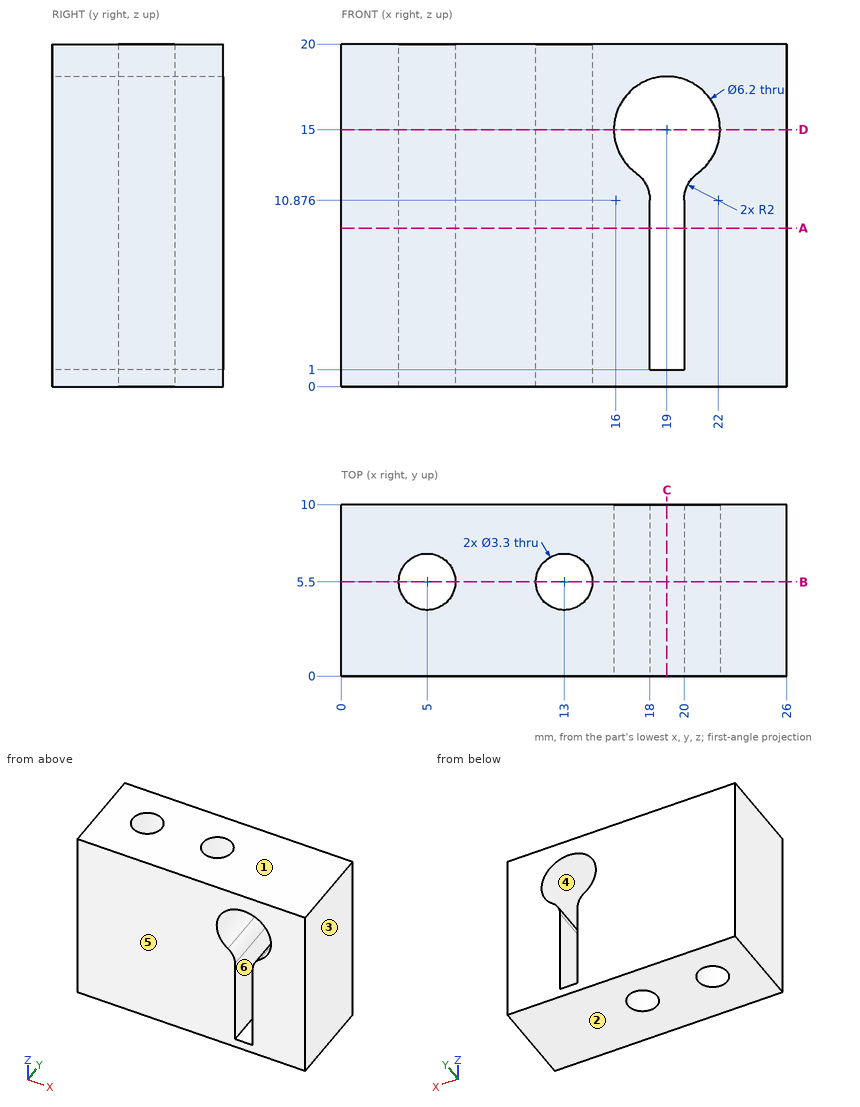
The figure shows three views and two pictorial views of one solid part (mm, origin at its lowest corner). Answer the questions. A direction names the side the tool comes from. Round coordinates to 2 decimals unless told otherwise and drop trailing zeros. Write each loop counter-clockwise with the first axis right and the second up, starting at its lowest first coordinate (ties: lowest second). Pieces come first, ordered by that corner, then holes. Notation, with made-up numbers: (-3.75, -24.5) -> (37.25, -24.5) arc R13 ccw to (37.25, -2.5) -> close; hole circle Ø9 at (51, -12). An arc over 180 degrees is marked (long way). Answer as a JSON object with one key per item and string values. Group by question number.
Q1. Determine the mould class of the marked faces 1, 2, 3 and 4 for opening direction Z: pulls with the +Z half, pulls with the -Z half, needs draft (parallel to the pull), parting line crosses it, or undercut.
Q2. Section A-A (z = 9.25) is taken. Write down the section's boundary in (x, y), plus the area to 3 significant figures.
Q3. Section B-B (y = 5.5) is taken. Write down the section's boundary in (x, z).
Q4. Section C-C (x = 19) is taken. Write down the section's boundary in (y, z).
Q5. Which of the six approach directions +Z, -Z, +X, -X, +Y, -Y give full straight-line access (tool end or side, diameter ignored) to the marked faces 5 and 6?
Q6. Straight lines are drawn through the part: line 1 along Y through (x, z) = (5, 5.25); line 2 along X through (y, z) = (7.5, 4.25); line 3 along X through (y, z) = (6, 12) (1 decimal). For each, find the intervals that lie inside material, in ascending order.
Q7. Section D-D (z = 15) is taken. Write down the section's boundary in (x, y), plus the area to 3 significant figures.
Check values:
{
 "1": {"face 1": "pulls with the +Z half", "face 2": "pulls with the -Z half", "face 3": "needs draft", "face 4": "undercut"},
 "2": {"outline": "(0, 0) -> (18, 0) -> (18, 10) -> (0, 10) -> close; (20, 0) -> (26, 0) -> (26, 10) -> (20, 10) -> close; hole circle Ø3.3 at (5, 5.5); hole circle Ø3.3 at (13, 5.5)", "area": "223 mm^2"},
 "3": {"outline": "(0, 0) -> (3.35, 0) -> (3.35, 20) -> (0, 20) -> close; (6.65, 0) -> (11.35, 0) -> (11.35, 20) -> (6.65, 20) -> close; (14.65, 0) -> (26, 0) -> (26, 20) -> (14.65, 20) -> close; hole (17.18, 12.49) arc R2 cw to (18, 10.88) -> (18, 1) -> (20, 1) -> (20, 10.88) arc R2 cw to (20.82, 12.49) arc R3.1 ccw (long way) to start"},
 "4": {"outline": "(0, 0) -> (10, 0) -> (10, 1) -> (0, 1) -> close; (0, 18.1) -> (10, 18.1) -> (10, 20) -> (0, 20) -> close"},
 "5": {"face 5": "+Z, -Z, +X, -X, -Y", "face 6": "+Y, -Y"},
 "6": {"line 1": "0 to 3.85, 7.15 to 10", "line 2": "0 to 18, 20 to 26", "line 3": "0 to 3.4, 6.6 to 11.4, 14.6 to 17.7, 20.3 to 26"},
 "7": {"outline": "(0, 0) -> (15.9, 0) -> (15.9, 10) -> (0, 10) -> close; (22.1, 0) -> (26, 0) -> (26, 10) -> (22.1, 10) -> close; hole circle Ø3.3 at (5, 5.5); hole circle Ø3.3 at (13, 5.5)", "area": "181 mm^2"}
}
